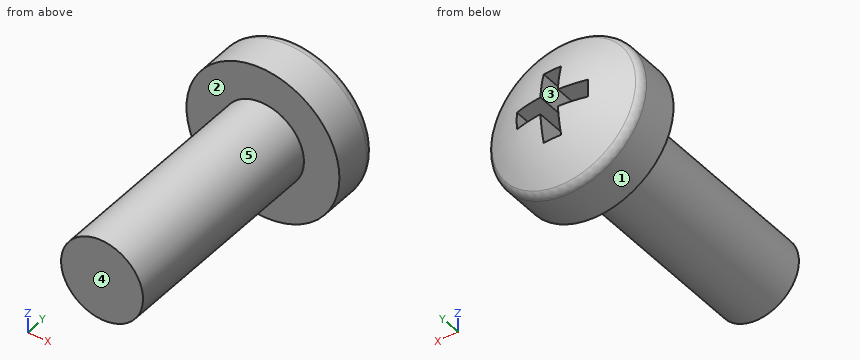
```python
from build123d import *

# Parameters (mm, degrees)
SKETCH2_R           = 1.5
BOSS_EXTRUDE2_DEPTH = 8
CUT_EXTRUDE1_REACH  = 11.504
FILLET1_R           = 0.36


with BuildPart() as part:
    # Boss-Extrude1: read off the stored shape, not the designer's step
    # Boss-Extrude1 outline → Boss-Extrude1 (revolve)
    with BuildSketch(Plane.XY):
        with BuildLine():
            Line((2.8, 0), (2.8, 1.542463035))
            ThreePointArc((2.8, 1.542463035), (1.464186604, 2.180811394), (0, 2.4))
            Line((0, 2.4), (0, 0))
            Line((0, 0), (2.8, 0))
        make_face()
    revolve(axis=Axis((0, 0, 0), (0, 1, 0)))

    # Sketch2 → Boss-Extrude2 (add)
    with BuildSketch(Plane.XZ):
        with Locations(Location((0, 0, 0), (0, 0, 270))):
            Circle(SKETCH2_R)
    extrude(amount=BOSS_EXTRUDE2_DEPTH)

    # Sketch3 → Cut-Extrude1 (cut, up to next)
    with BuildSketch(Plane.XZ.offset(-0.64), mode=Mode.PRIVATE) as cut_extrude1_sk1:
        Polygon((-0.32, -1.3), (0.32, -1.3), (0.32, -0.32), (1.3, -0.32), (1.3, 0.32), (0.32, 0.32), (0.32, 1.3), (-0.32, 1.3), (-0.32, 0.32), (-1.3, 0.32), (-1.3, -0.32), (-0.32, -0.32), align=None)
    cut_extrude1_tool1 = extrude(cut_extrude1_sk1.sketch, amount=-CUT_EXTRUDE1_REACH, mode=Mode.PRIVATE) & part.part
    add(cut_extrude1_tool1.solids().sort_by_distance((0, 0.64, 0))[0], mode=Mode.SUBTRACT)

    # Fillet1
    fillet1_edges = [part.edges().sort_by_distance(p)[0] for p in [
        (-2.8, 1.542463035, 0),
    ]]
    fillet(fillet1_edges, radius=FILLET1_R)


solid = part.part
```
The model under review builds one solid part; all positions refer to its coordinate system, in mm. Face numbers are marked on the shaded views. A direction names the side the tool comes from. Give positions to 0.01 mm unless a question says otherwise; leave off trailing zeros. Write each loop counter-clockwise with the first axis right and the second up, starting at its lowest first coordinate (ties: lowest second). Pieces come first, ordered by that corner, then holes. Notation, with made-up numbers: M -9,14 L 32,14 A8 cw 32,20 Z; hole C 78,53.5 d5. An arc over 180 degrees is marked long. Write each question's results on one line, items separated by ' | '. Start each with the question number.
1. Mouldability with a two-part tool opening along Z and no side actions: class the marked faces 3, 4 and 5 as released by +Z, released by -Z, zero draft, split by the parting line, or undercut.
2. For the marked faces 1 and 2, list the 3-axis set-ups (+Z, -Z, +X, -X, +Y, -Y) from which the entire face can be reached by the end or side of a thin tool; tool diameter is ignored.
3. We need section A-A (y = -2). Write out the cut boundary in (x, z), and give its area (3 significant figures).
4. For probe 1 along Z at (x, y) = (-0.55, 1); probe 2 along Z at (x, y) = (1.25, 1); probe 3 along X at (y, z) = (1.5, 0.5), list the stretches that pass through material, from the lowest coordinate up. Write a range as [from, to].
5. Insertion check: pin 1 Ø0.5 at (x, y) = (-1, 1) entering from -Z; pin 2 Ø1.1 at (y, z) = (2, -0.5) entering from -X; pin 3 Ø0.8 at (y, z) = (1.5, 0.5) entering from +X. Each pin has a flat end and moves straight along its axis. Give the tip position at first contact, or say it passes through.
Results found:
1) face 3: undercut | face 4: zero draft | face 5: split by the parting line
2) face 1: +Y, -Y | face 2: -Y
3) outline: C 0,0 d3 | area: 7.07 mm^2
4) probe 1: z = [-2.75, -0.32], [0.32, 2.75] | probe 2: z = [-2.51, -0.32], [0.32, 2.51] | probe 3: x = [-2.72, -0.32], [0.32, 2.72]
5) pin 1: stops at z = -2.7 | pin 2: stops at x = -2.76 | pin 3: stops at x = 2.8
